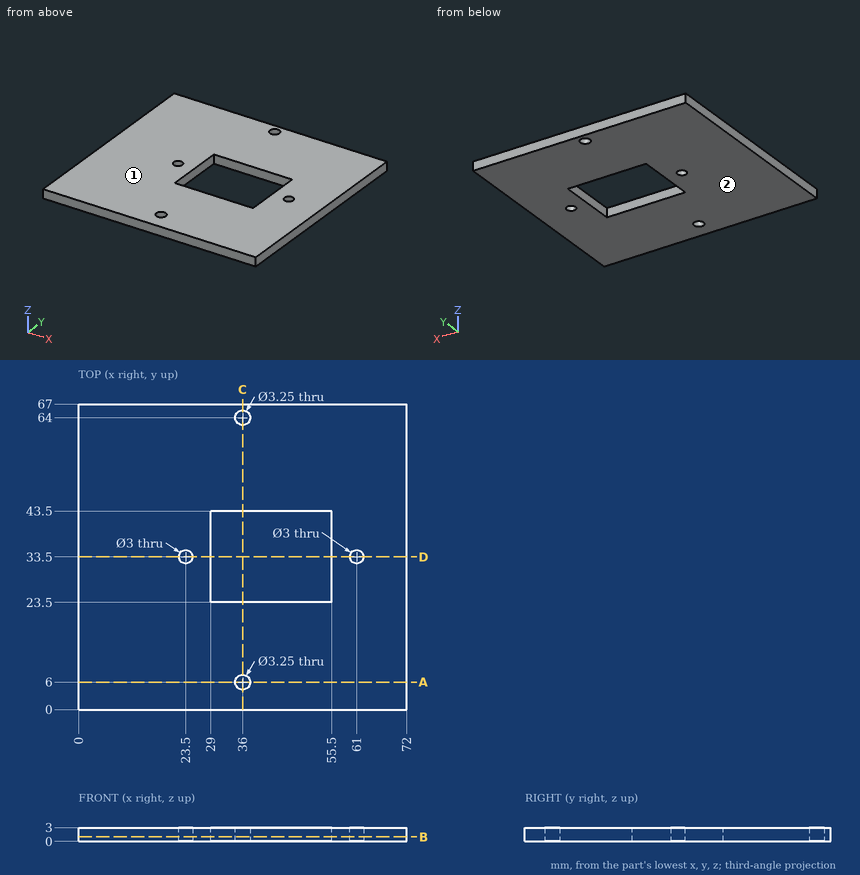
Print and shaded views of the part. All mm, measured from the part's lowest x, y and z. Give positions to 0.01 mm unless a question says otherwise; leave off trailing zeros. Loops run counter-clockwise (first coordinate to the right, second up) from the corner with the lowest first, then second, coordinate; pieces in that order, holes last.
1) Saw through at B-B (z = 0.95). Write the cut outline in (x, y) (3 decimals).
2) Saw through at A-A (y = 6). Write the cut outline in (x, z) (3 decimals).
3) Pull direction Z, two halves, no side cores. Call the marked faces 1 and 2: +Z half, -Z half, draft (parallel to the pull), parting line (faces both ways), or undercut.
4) Saw through at C-C (x = 36). Write the cut outline in (y, z) (3 decimals).
5) Saw through at D-D (y = 33.5). Write the cut outline in (x, z), plus the area to 4 significant figures.
6) Wall check: line 1 (Y direction, x = 36, z = 1.3) (3 decimals); line 2 (X direction, y = 39, z = 0.6); line 3 (Y direction, x = 61, z = 2.25). Give the ranges that are in metal, low to high.
7) Flat gauge pin, fed straight in: pin 1 Ø3 at (x, y) = (36, 6) entering from +Z. Where does the tip first touch, or does it go through?
Answer block:
1. outline: (0, 0) - (72, 0) - (72, 67) - (0, 67) - close; hole circle Ø3 at (23.5, 33.5); hole (29, 23.5) - (55.5, 23.5) - (55.5, 43.5) - (29, 43.5) - close; hole circle Ø3.25 at (36, 6); hole circle Ø3.25 at (36, 64); hole circle Ø3 at (61, 33.5)
2. outline: (0, 0) - (34.375, 0) - (34.375, 3) - (0, 3) - close; (37.625, 0) - (72, 0) - (72, 3) - (37.625, 3) - close
3. face 1: +Z half
3. face 2: -Z half
4. outline: (0, 0) - (4.375, 0) - (4.375, 3) - (0, 3) - close; (7.625, 0) - (23.5, 0) - (23.5, 3) - (7.625, 3) - close; (43.5, 0) - (62.375, 0) - (62.375, 3) - (43.5, 3) - close; (65.625, 0) - (67, 0) - (67, 3) - (65.625, 3) - close
5. outline: (0, 0) - (22, 0) - (22, 3) - (0, 3) - close; (25, 0) - (29, 0) - (29, 3) - (25, 3) - close; (55.5, 0) - (59.5, 0) - (59.5, 3) - (55.5, 3) - close; (62.5, 0) - (72, 0) - (72, 3) - (62.5, 3) - close
5. area: 118.5 mm2
6. line 1: y = 0 to 4.375, 7.625 to 23.5, 43.5 to 62.375, 65.625 to 67
6. line 2: x = 0 to 29, 55.5 to 72
6. line 3: y = 0 to 32, 35 to 67
7. pin 1: passes through
